from build123d import *

# Parameters (mm, degrees)
BOSS_EXTRUDE1_DEPTH = 19
SKETCH2_W           = 24
SKETCH2_H           = 15
CUT_EXTRUDE1_DEPTH  = 38.59555024
SKETCH3_W           = 5.291502622
SKETCH3_H           = 15
CUT_EXTRUDE2_DEPTH  = 39.990548382
SKETCH4_R           = 3.1
CUT_EXTRUDE4_DEPTH  = 9


with BuildPart() as part:
    # Sketch1 → Boss-Extrude1 (new body)
    with BuildSketch(Plane(origin=(0, 0, 0), x_dir=(1, 0, 0), z_dir=(0, 1, 0))):
        with BuildLine():
            Line((16.383693046, 8.628297362), (-11.616306954, 8.628297362))
            Line((-11.616306954, 8.628297362), (-11.616306954, -11.371702638))
            ThreePointArc((-11.616306954, -11.371702638), (-5.185236036, -19.216348043), (3.76830843, -14.448625715))
            ThreePointArc((3.76830843, -14.448625715), (5.610192064, -12.211451166), (8.383693046, -11.371702638))
            Line((8.383693046, -11.371702638), (15.383693046, -11.371702638))
            ThreePointArc((15.383693046, -11.371702638), (16.090799827, -11.078809419), (16.383693046, -10.371702638))
            Line((16.383693046, -10.371702638), (16.383693046, 8.628297362))
        make_face()
        with BuildLine():
            ThreePointArc((-7.766306954, -11.371702638), (-3.616306954, -15.521702638), (0.533693046, -11.371702638))
            ThreePointArc((0.533693046, -11.371702638), (-3.616306954, -7.221702638), (-7.766306954, -11.371702638))
        make_face(mode=Mode.SUBTRACT)
    extrude(amount=BOSS_EXTRUDE1_DEPTH)

    # Sketch2 → Cut-Extrude1 (cut, through all)
    with BuildSketch(Plane(origin=(0, 0, -8.628297362), x_dir=(-1, 0, 0), z_dir=(0, 0, -1))):
        with Locations((-2.383693046, 9.5)):
            Rectangle(SKETCH2_W, SKETCH2_H)
    extrude(amount=-CUT_EXTRUDE1_DEPTH, mode=Mode.SUBTRACT)

    # Sketch3 → Cut-Extrude2 (cut, through all)
    with BuildSketch(Plane.ZY.offset(11.616306954)):
        with Locations((14.017453949, 9.5)):
            Rectangle(SKETCH3_W, SKETCH3_H)
    extrude(amount=-CUT_EXTRUDE2_DEPTH, mode=Mode.SUBTRACT)

    # Sketch4 → Cut-Extrude4 (cut)
    with BuildSketch(Plane(origin=(16.383693046, 0, 0), x_dir=(0, 0, -1), z_dir=(1, 0, 0))):
        with Locations((1.628297362, 9.5)):
            Circle(SKETCH4_R)
    extrude(amount=-CUT_EXTRUDE4_DEPTH, mode=Mode.SUBTRACT)


solid = part.part
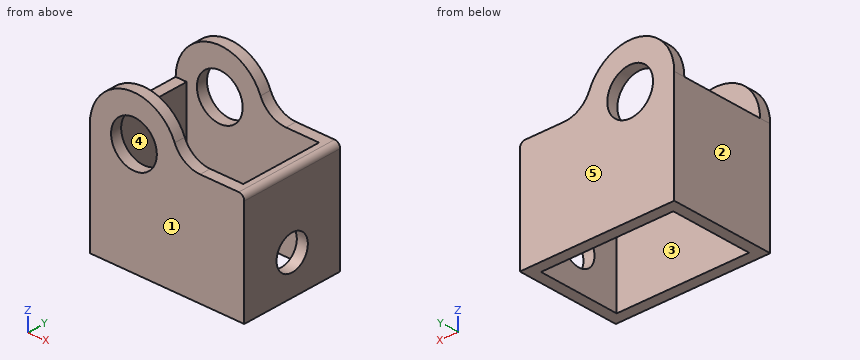
Geometry: final body of the model. Coordinates: model frame, mm. Face numbers are marked on the shaded views. A direction names the side the tool comes from. Give positions to 0.01 mm unless a question says otherwise; leave off trailing zeros. Order: outer loops, then holes, each group sorted by start corner. A loop starts at its lowest first (then second) coordinate and runs counter-clockwise, first axis right, second up. Notation, with made-up numbers: (27, 42) -> (66, 42) arc R5 cw to (66, 49) -> close; hole circle Ø9 at (38, 33.5). An arc over 180 degrees is marked (long way). Put each result on its own line as item: value.
Q1. Reachability of the marked faces 4 and 5 from +Z, -Z, +X, -X, +Y, -Y: full face, straight path, thin tool, end or side. Return the list, or none.
Here are the results:
face 4: +Z, -Z
face 5: +Z, -Z, +X, -X, +Y
Q2. Section C-C, the plane y = 15. Return loops of the section in (x, z).
Here are the results:
outline: (-11.62, -8.63) -> (-9.62, -8.63) -> (-9.62, 11.37) -> (-11.62, 11.37) -> close; (14.38, -8.63) -> (16.38, -8.63) -> (16.38, 10.37) arc R1 ccw to (15.38, 11.37) -> (14.38, 11.37) -> close
Q3. Pin query (flat end, axial travel): pin 1 (3.5 mm diameter, centred on y = 9.5, z = -1.63, fed in from +X); pin 2 (1 mm diameter, centred on x = -11, y = 10, fed in from +Z). Return the tip coordinate at first contact, or that it passes through.
Here are the results:
pin 1: stops at x = -9.62
pin 2: stops at z = 11.37
Q4. Draft query along X for the marked faces 1, 2 and 3. Return one class per face: released by +X, released by -X, zero draft, split by the parting line, or undercut.
Here are the results:
face 1: zero draft
face 2: released by -X
face 3: undercut
Q5. Section A-A, the plane y = 9.5. Return loops of the section in (x, z), then the cut area to 3 significant figures.
Here are the results:
outline: (-11.62, -8.63) -> (-9.62, -8.63) -> (-9.62, 11.37) -> (-11.62, 11.37) -> close; (14.38, -8.63) -> (16.38, -8.63) -> (16.38, -4.73) -> (14.38, -4.73) -> close; (14.38, 1.47) -> (16.38, 1.47) -> (16.38, 10.37) arc R1 ccw to (15.38, 11.37) -> (14.38, 11.37) -> close
area: 67.4 mm^2
Q6. Section D-D, the plane x = 7.5. Return loops of the section in (y, z).
Here are the results:
outline: (0, -8.63) -> (2, -8.63) -> (2, 11.45) -> (0, 11.45) -> close; (17, -8.63) -> (19, -8.63) -> (19, 11.45) -> (17, 11.45) -> close
Q7. Material intervals for L1, parallel to X at y = 2.25, z = -5.75; L2, parallel to Y at x = 10, z = 9.75; L3, parallel to X at y = 10.25, z = -0.25, sorted ascending.
Here are the results:
L1: x = -11.62 to -9.62, 14.38 to 16.38
L2: y = 0 to 2, 17 to 19
L3: x = -11.62 to -9.62
Q8. Section B-B, the plane z = -6. Return loops of the section in (x, y), then the cut area to 3 significant figures.
Here are the results:
outline: (-11.62, 0) -> (16.38, 0) -> (16.38, 19) -> (-11.62, 19) -> close; hole (-9.62, 2) -> (14.38, 2) -> (14.38, 17) -> (-9.62, 17) -> close
area: 172 mm^2
